Autodesk Inventor part; units mm, degrees
ref_plane "作業平面1" through (0, 0, 148.47) normal (0, 0, -1) x (-1, 0, 0)
ref_plane "作業平面2" through (10.5, -15, 148.47) normal (0, 1, 0) x (-1, 0, 0)
ref_plane "YZ Plane" through (0, 0, 0) normal (1, 0, 0) x (0, 1, 0)
sketch "スケッチ1" plane through (0, 0, 0) normal (0, 0, 1) x (1, 0, 0)
  circle A0 centre (0, 0) radius 8
  dimension "d0" = 16
extrude "押し出し1" add sketch "スケッチ1" along normal blind 88.47
sketch "スケッチ2" plane through (0, 0, 0) normal (0, 0, -1) x (-1, 0, 0)
  point P0 (0, 0)
  point P1 (0, 0)
sketch "スケッチ3" plane through (0, 0, 88.47) normal (0, 0, 1) x (1, 0, 0)
  circle A0 centre (0, 0) radius 10.5
  dimension "d4" = 21
extrude "押し出し2" add sketch "スケッチ3" along normal blind 82
fillet "フィレット1" radius 8 1 edges at (-8, 0, 0)
sketch "スケッチ4" plane through (0, 0, 0) normal (0, 1, 0) x (-1, 0, 0)
  circle A0 centre (0, 170.47) radius 20
  line L0 (10.5, 170.47) -> (-10.5, 170.47)
  point P0 (0, 0)
  dimension "d7" = 40
  dimension "d25" = 0
extrude "押し出し3" add sketch "スケッチ4" along normal mid plane 28
ref_plane "作業平面1" through (0, 0, 148.47) normal (0, 0, -1) x (-1, 0, 0)
sketch "スケッチ5" plane through (0, 0, 148.47) normal (0, 0, -1) x (-1, 0, 0)
  line L0 (10.5, 15) -> (-10.5, 15)
  line L1 (-10.5, 15) -> (-10.5, -15)
  line L2 (-10.5, -15) -> (10.5, -15)
  line L3 (10.5, -15) -> (10.5, 15)
  line L4 (10.5, 15) -> (-10.5, -15) construction
  line L5 (-10.5, 15) -> (10.5, -15) construction
  point P0 (0, 0)
  dimension "d11" = 21
  dimension "d12" = 30
ref_plane "作業平面2" through (10.5, -15, 148.47) normal (0, 1, 0) x (-1, 0, 0)
sketch "スケッチ8" plane through (10.5, -15, 148.47) normal (0, 1, 0) x (-1, 0, 0)
  circle A0 centre (10.5, 19.2998) radius 6.5
  point P0 (10.5, -148.47)
  dimension "d14" = 13
extrude "押し出し4" add sketch "スケッチ8" along normal mid plane 24
sketch "スケッチ9" plane through (0, -27, 167.7698) normal (0, -1, 0) x (1, 0, 0)
  circle A0 centre (0, 0) radius 5
  point P0 (0, -167.7698)
  dimension "d17" = 10
extrude "押し出し5" add sketch "スケッチ9" along normal blind 21
sketch "スケッチ11" plane through (0, 0, 0) normal (0, 0, 1) x (1, 0, 0)
  line L0 (-25, -25) -> (25, -25)
  line L1 (25, -25) -> (25, 25)
  line L2 (25, 25) -> (-25, 25)
  line L3 (-25, 25) -> (-25, -25)
  line L4 (-25, -25) -> (25, 25) construction
  line L5 (25, -25) -> (-25, 25) construction
  point P0 (0, 0)
  dimension "d23" = 50
  dimension "d24" = 50
properties part number "ラックアンドピニオンの左右の棒"
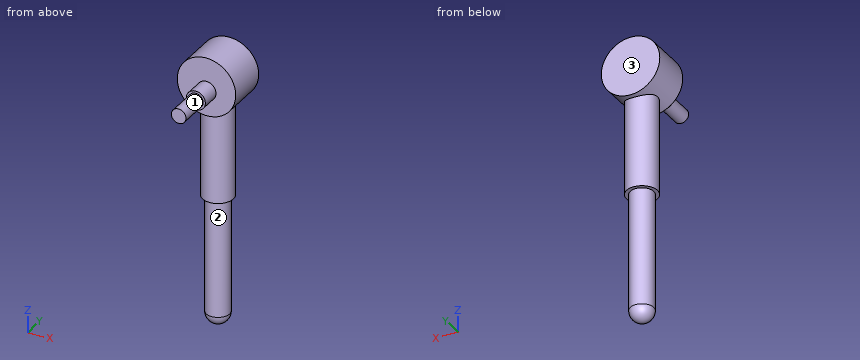
Check sheet for the modelled part. Datum: model origin and axes. Units: mm. Face numbers are marked on the shaded views. A direction names the side the tool comes from. Round coordinates to 2 decimals unless told otherwise and drop trailing zeros. Loops run counter-clockwise (first coordinate to the right, second up) from the corner with the lowest first, then second, coordinate; pieces in that order, holes last.
1. Set-up check for the marked faces 1, 2 and 3: record each of +Z, -Z, +X, -X, +Y, -Y from which the full face is reachable in a straight line by a thin tool's end or side.
2. Sectioned sample at A-A on y = 0. Record the boundary of the cut face in (x, z), and give its area (3 significant figures).
3. Sectioned sample at D-D on z = 170.47. Record the boundary of the cut face in (x, y), and give its area (3 significant figures).
4. Scan lines: probe 1 along Y at (x, z) = (-4, 159.5); probe 2 along Z at (x, y) = (-0.5, -25.5); probe 3 along X at (y, z) = (-10, 162.5). Record each from-to range of solid material in increasing order.
5. Sectioned sample at B-B on x = 0. Record the boundary of the cut face in (y, z).
6. Sectioned sample at C-C on z = 47.5. Record the boundary of the cut face in (x, y), and give its area (3 significant figures).
7. Gauge pin test, flat ends, axial feed: pin 1 Ø3 at (x, y) = (5, -22) entering from +Z; pin 2 Ø10 at (x, z) = (14, 164) entering from -Y; pin 3 Ø12 at (x, y) = (15, -13) entering from -Z. Record the tip position at first contact, or that the pin passes through.
Recorded:
1. face 1: -Y
1. face 2: -Z
1. face 3: +Z, -Z, +X, -X, +Y
2. outline: (-10.5, 88.47) - (-8, 88.47) - (-8, 8) arc R8 ccw to (8, 8) - (8, 88.47) - (10.5, 88.47) - (10.5, 153.45) arc R20 ccw (long way) to (-10.5, 153.45) - close
2. area: 3,970 mm2
3. outline: (-20, -14) - (-5.91, -14) - (-5.91, -27) - (-4.21, -27) - (-4.21, -48) - (4.21, -48) - (4.21, -27) - (5.91, -27) - (5.91, -14) - (20, -14) - (20, 14) - (-20, 14) - close
3. area: 1,450 mm2
4. probe 1: y = -14 to 14
4. probe 2: z = 161.29 to 174.25
4. probe 3: x = -18.34 to 18.34
5. outline: (-48, 162.77) - (-27, 162.77) - (-27, 161.27) - (-14, 161.27) - (-14, 150.47) - (-10.5, 150.47) - (-10.5, 88.47) - (-8, 88.47) - (-8, 8) arc R8 ccw to (8, 8) - (8, 88.47) - (10.5, 88.47) - (10.5, 150.47) - (14, 150.47) - (14, 190.47) - (-14, 190.47) - (-14, 174.27) - (-27, 174.27) - (-27, 172.77) - (-48, 172.77) - close
6. outline: circle Ø16 at (0, 0)
6. area: 201 mm2
7. pin 1: stops at z = 173.25
7. pin 2: stops at y = -14
7. pin 3: stops at z = 152.61
